```python
from build123d import *

# Parameters (mm, degrees)
F1_DEPTH = 63.5
F2_DEPTH = 25.4
F3_DEPTH = 12.7
F5_R     = 6.35


with BuildPart() as f1:
    # F0 (on Front) → F1 (new body, symmetric)
    with BuildSketch(Plane.XZ):
        Polygon((22.225, 9.525), (-41.275, 9.525), (-41.275, -9.525), (41.275, -9.525), (41.275, 9.525), align=None)
    extrude(amount=F1_DEPTH, both=True)

    # F0 (on Front) → F2 (join, symmetric)
    with BuildSketch(Plane.XZ):
        with BuildLine():
            Line((22.225, 24.7660442862), (22.225, 9.525))
            Line((22.225, 9.525), (41.275, 9.525))
            Line((41.275, 9.525), (41.275, 24.7660442862))
            ThreePointArc((41.275, 24.7660442862), (46.8632744023, 38.1864149015), (60.325, 43.6743199825))
            Line((60.325, 43.6743199825), (60.325, 62.7245845587))
            add(Edge.make_bspline(
                [(58.6218546558, 62.6926976316), (59.1901148173, 62.7069385572), (59.7578604016, 62.7175822247), (60.325, 62.7245845587)],
                knots=[113.3285433614, 113.3285433614, 113.3285433614, 113.3285433614, 114.6854646292, 114.6854646292, 114.6854646292, 114.6854646292], degree=3))
            ThreePointArc((58.6218546558, 62.6926976316), (32.7962107912, 51.0489382613), (22.225, 24.7660442862))
        make_face()
        Polygon((60.325, 66.675), (60.325, 62.7245845587), (60.325, 43.6743199825), (85.5901753482, 43.6743199825), (85.0338637829, 66.675), align=None)
        Polygon((85.5901753482, 43.6743199825), (60.325, 43.6743199825), (60.325, 38.1), (85.725, 38.1), align=None)
    extrude(amount=F2_DEPTH, both=True)

    # F0 (on Front) → F3 (join, symmetric)
    with BuildSketch(Plane.XZ):
        with BuildLine():
            add(Edge.make_bspline(
                [(-41.275, 9.525), (-39.8884323403, 35.2216003411), (11.1614029089, 61.5033114907), (58.6218546558, 62.6926976316)],
                knots=[0, 0, 0, 0, 113.3285433614, 113.3285433614, 113.3285433614, 113.3285433614], degree=3))
            Line((-41.275, 9.525), (22.225, 9.525))
            Line((22.225, 9.525), (22.225, 24.7660442862))
            ThreePointArc((22.225, 24.7660442862), (32.7962107912, 51.0489382613), (58.6218546558, 62.6926976316))
        make_face()
    extrude(amount=F3_DEPTH, both=True)

    # F0 (on Front) → F4 (revolve)
    with BuildSketch(Plane.XZ):
        Polygon((85.0338637829, 66.675), (85.5901753482, 43.6743199825), (85.725, 38.1), (111.125, 38.1), (111.125, 66.675), align=None)
    revolve(axis=Axis((85.3794318914, 0, 52.3875), (-0.0241796728, 0, 0.999707629)))

    # F5
    f5_edges = [f1.edges().sort_by_distance(p)[0] for p in [
        (-41.275, -63.5, 0),
        (41.275, -63.5, 0),
        (-41.275, 63.5, 0),
        (41.275, 63.5, 0),
    ]]
    fillet(f5_edges, radius=F5_R)


solid = f1.part
```
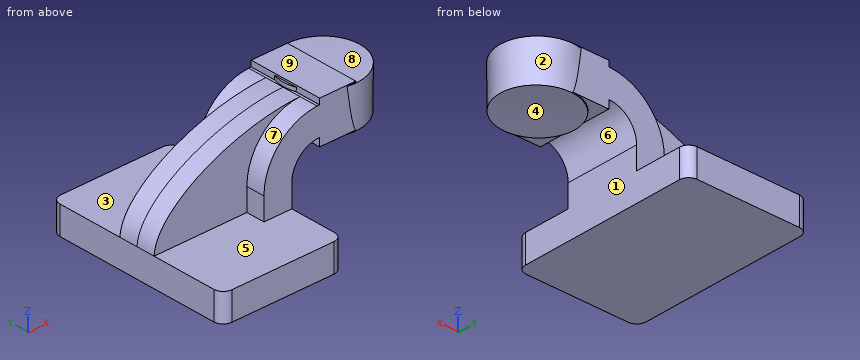
Can you work these out from the model? Positions are in its coordinate system, mm. Face numbers are marked on the shaded views. A direction names the side the tool comes from. Round coordinates to 2 decimals unless told otherwise and drop trailing zeros. Loops run counter-clockwise (first coordinate to the right, second up) from the corner with the lowest first, then second, coordinate; pieces in that order, holes last. Notation, with made-up numbers: M 7.5,-37.75 L 43.5,-37.75 A9 cw 43.5,-31.75 Z; hole C 76.25,-11 d10. An arc over 180 degrees is marked long. Answer in a Markdown table with one row per item.
1. On a 3-axis mill with a long thin cutter (end or side, diameter ignored), from which of +Z, -Z, +X, -X, +Y, -Y can I reach the whole of each face in a straight line? I mean the marked faces 1, 2, 3, 4 and 5. Say none if no direction works.
Established:
| item | result |
|---|---|
| face 1 | -Z, +X, +Y, -Y |
| face 2 | -Z |
| face 3 | +Z, -X, +Y |
| face 4 | -Z, +X |
| face 5 | +Z, -X, -Y |
2. Please list where these lines run through material, in increasing order: line 1 (Z direction, x = -15, y = 50) (3 decimals); line 2 (Y direction, x = 81.5, z = 42.5); line 3 (X direction, y = -35.5, z = -3.5) (3 decimals). Write a range as from..to.
Established:
| item | result |
|---|---|
| line 1 | -9.525..9.525 |
| line 2 | -25.4..25.4 |
| line 3 | -41.275..41.275 |
3. If we section it at B-B, the plane y = 36: Please give me the cut outline in (x, z) (3 decimals), plus the area to 3 significant figures.
Established:
| item | result |
|---|---|
| outline | M -41.275,-9.525 L 41.275,-9.525 L 41.275,9.525 L -41.275,9.525 Z |
| area | 1,570 mm² |
4. If we section it at A-A, the plane z = -2: Please give me the cut outline in (x, y) (3 decimals).
Established:
| item | result |
|---|---|
| outline | M -41.275,-57.15 A6.35 ccw -34.925,-63.5 L 34.925,-63.5 A6.35 ccw 41.275,-57.15 L 41.275,57.15 A6.35 ccw 34.925,63.5 L -34.925,63.5 A6.35 ccw -41.275,57.15 Z |
5. Thinking about a two-plate mould opening in X: for the marked faces 6, 7, 8 and 9, which applies, pulls with the +X half, pulls with the -X half, needs draft (parallel to the pull), parting line crosses it, or undercut?
Established:
| item | result |
|---|---|
| face 6 | undercut |
| face 7 | pulls with the -X half |
| face 8 | undercut |
| face 9 | needs draft |
6. I'm going to push flat-ended pins straight in: pin 1 Ø2 at (y, z) = (9.5, 47.5) entering from +X; pin 2 Ø1.7 at (y, z) = (-10.5, 40.5) entering from -X; pin 3 Ø10.5 at (y, z) = (-15.5, 3.5) entering from +X (3 decimals). Where does each tip first touch, or does it pass through?
Established:
| item | result |
|---|---|
| pin 1 | x = 109.67 |
| pin 2 | x = -18.21 |
| pin 3 | x = 41.275 |
